Input: part model. Units: mm. Frame: model coordinates. A direction names the side the tool comes from. Round coordinates to 2 decimals unless told otherwise and drop trailing zeros. Loops run counter-clockwise (first coordinate to the right, second up) from the corner with the lowest first, then second, coordinate; pieces in that order, holes last.
(1) Cut plane D-D, the plane z = 18. Output: boundary loops of the cut face in (x, y), and give its area (3 significant figures).
(2) Access query for faces 4 (the face through (-55, 114, 0)), 5 (the face through (1.352, 222.535, 4.292)), 6 (the face through (-1, 220, 6)). Directions: +Z, -Z, +X, -X, +Y, -Y. A direction counts if a zero-diameter tool reaches every point of the face in a straight line with its end or side. Return the directions, or none.
(3) Cut plane B-B, the plane x = -68. Output: boundary loops of the cut face in (y, z).
(4) Cut plane A-A, the plane y = 135.5. Output: boundary loops of the cut face in (x, z).
(5) Line query: line 1 (X direction, y = 81, z = -1.5); line 2 (X direction, y = 222, z = 0); line 3 (Z direction, x = 68, y = 3.5). Output: solid intervals per line, ascending.
(6) Draft query along X for faces 1 (the face through (-63, 0, 0)), 2 (the face through (55, 111, 0)), 3 (the face through (-51.804, 1.711, 0.35)). Return one class per face: released by +X, released by -X, zero draft, split by the parting line, or undercut.
(7) First-contact query: pin 1 Ø25 at (y, z) = (92.5, -3) entering from -X; pin 2 Ø4 at (y, z) = (88, -11) entering from +X; pin 3 Ø19 at (x, z) = (64, 12.5) entering from +Y; pin 4 Ø8 at (x, z) = (68, 0) entering from -Y. Flat tips, straight axial feed; report the tip coordinate or a pass-through.
(8) Cut plane C-C, the plane z = 0. Give the number of separate pieces and of enclosed holes in the cut face, and give its area (3 significant figures).
from build123d import *

# Parameters (mm, degrees)
BASE_FLANGE1_DEPTH = 25
CUT_EXTRUDE1_REACH = 237.425
SKETCH7_R          = 3
CUT_EXTRUDE2_REACH = 242.104
SKETCH8_R          = 4.5
FILLET1_R          = 3


# Sheet-metal steps are written as plain solids
with BuildPart() as part:
    # Sketch1 → Base-Flange1 (new, symmetric)
    with BuildSketch(Plane.XY):
        with BuildLine():
            Line((-80, 0), (-56, 0))
            ThreePointArc((-56, 0), (-51.757359313, 1.757359313), (-50, 6))
            Line((-50, 6), (-50, 219))
            ThreePointArc((-50, 219), (-49.707106781, 219.707106781), (-49, 220))
            Line((-49, 220), (49, 220))
            ThreePointArc((49, 220), (49.707106781, 219.707106781), (50, 219))
            Line((50, 219), (50, 6))
            ThreePointArc((50, 6), (51.757359313, 1.757359313), (56, 0))
            Line((56, 0), (80, 0))
            Line((80, 0), (80, 5))
            Line((80, 5), (56, 5))
            ThreePointArc((56, 5), (55.292893219, 5.292893219), (55, 6))
            Line((55, 6), (55, 219))
            ThreePointArc((55, 219), (53.242640687, 223.242640687), (49, 225))
            Line((49, 225), (-49, 225))
            ThreePointArc((-49, 225), (-53.242640687, 223.242640687), (-55, 219))
            Line((-55, 219), (-55, 6))
            ThreePointArc((-55, 6), (-55.292893219, 5.292893219), (-56, 5))
            Line((-56, 5), (-80, 5))
            Line((-80, 5), (-80, 0))
        make_face()
    extrude(amount=BASE_FLANGE1_DEPTH, both=True)

    # Sketch7 → Cut-Extrude1 (cut, up to next)
    with BuildSketch(Plane(origin=(0, 5, 0), x_dir=(1, 0, 0), z_dir=(0, 1, 0)), mode=Mode.PRIVATE) as cut_extrude1_sk1:
        with Locations(Location((68, 0, 0), (0, 0, 180))):
            Circle(SKETCH7_R)
    cut_extrude1_tool1 = extrude(cut_extrude1_sk1.sketch, amount=-CUT_EXTRUDE1_REACH, mode=Mode.PRIVATE) & part.part
    # Sketch7 → Cut-Extrude1 (cut, up to next)
    with BuildSketch(Plane(origin=(0, 5, 0), x_dir=(1, 0, 0), z_dir=(0, 1, 0)), mode=Mode.PRIVATE) as cut_extrude1_sk2:
        with Locations(Location((-68, 0, 0), (0, 0, 180))):
            Circle(SKETCH7_R)
    cut_extrude1_tool2 = extrude(cut_extrude1_sk2.sketch, amount=-CUT_EXTRUDE1_REACH, mode=Mode.PRIVATE) & part.part
    add(cut_extrude1_tool1.solids().sort_by_distance((68, 5, 0))[0], mode=Mode.SUBTRACT)
    add(cut_extrude1_tool2.solids().sort_by_distance((-68, 5, 0))[0], mode=Mode.SUBTRACT)

    # Sketch8 → Cut-Extrude2 (cut, up to next)
    with BuildSketch(Plane(origin=(0, 225, 0), x_dir=(1, 0, 0), z_dir=(0, 1, 0)), mode=Mode.PRIVATE) as cut_extrude2_sk1:
        with Locations(Location((0, 0, 0), (0, 0, 270))):
            Circle(SKETCH8_R)
    cut_extrude2_tool1 = extrude(cut_extrude2_sk1.sketch, amount=-CUT_EXTRUDE2_REACH, mode=Mode.PRIVATE) & part.part
    # Sketch8 → Cut-Extrude2 (cut, up to next)
    with BuildSketch(Plane(origin=(0, 225, 0), x_dir=(1, 0, 0), z_dir=(0, 1, 0)), mode=Mode.PRIVATE) as cut_extrude2_sk2:
        with Locations(Location((-25, 0, 0), (0, 0, 270))):
            Circle(SKETCH8_R)
    cut_extrude2_tool2 = extrude(cut_extrude2_sk2.sketch, amount=-CUT_EXTRUDE2_REACH, mode=Mode.PRIVATE) & part.part
    # Sketch8 → Cut-Extrude2 (cut, up to next)
    with BuildSketch(Plane(origin=(0, 225, 0), x_dir=(1, 0, 0), z_dir=(0, 1, 0)), mode=Mode.PRIVATE) as cut_extrude2_sk3:
        with Locations(Location((25, 0, 0), (0, 0, 270))):
            Circle(SKETCH8_R)
    cut_extrude2_tool3 = extrude(cut_extrude2_sk3.sketch, amount=-CUT_EXTRUDE2_REACH, mode=Mode.PRIVATE) & part.part
    add(cut_extrude2_tool1.solids().sort_by_distance((0, 225, 0))[0], mode=Mode.SUBTRACT)
    add(cut_extrude2_tool2.solids().sort_by_distance((-25, 225, 0))[0], mode=Mode.SUBTRACT)
    add(cut_extrude2_tool3.solids().sort_by_distance((25, 225, 0))[0], mode=Mode.SUBTRACT)

    # Fillet1
    fillet1_edges = [part.edges().sort_by_distance(p)[0] for p in [
        (80, 2.5, -25),
        (-80, 2.5, -25),
        (80, 2.5, 25),
        (-80, 2.5, 25),
    ]]
    fillet(fillet1_edges, radius=FILLET1_R)


solid = part.part
Reported:
1. outline: (-80, 0) - (-56, 0) arc R6 ccw to (-50, 6) - (-50, 219) arc R1 cw to (-49, 220) - (49, 220) arc R1 cw to (50, 219) - (50, 6) arc R6 ccw to (56, 0) - (80, 0) - (80, 5) - (56, 5) arc R1 cw to (55, 6) - (55, 219) arc R6 ccw to (49, 225) - (-49, 225) arc R6 ccw to (-55, 219) - (-55, 6) arc R1 cw to (-56, 5) - (-80, 5) - close
1. area: 2,970 mm2
2. face 4: +Z, -Z, -X, +Y
2. face 5: +Y, -Y
2. face 6: +Z, -Z, -Y
3. outline: (0, -25) - (5, -25) - (5, -3) - (0, -3) - close; (0, 3) - (5, 3) - (5, 25) - (0, 25) - close
4. outline: (-55, -25) - (-50, -25) - (-50, 25) - (-55, 25) - close; (50, -25) - (55, -25) - (55, 25) - (50, 25) - close
5. line 1: x = -55 to -50, 50 to 55
5. line 2: x = -54.2 to -29.5, -20.5 to -4.5, 4.5 to 20.5, 29.5 to 54.2
5. line 3: z = -25 to -3, 3 to 25
6. face 1: zero draft
6. face 2: released by +X
6. face 3: undercut
7. pin 1: stops at x = -55
7. pin 2: stops at x = 55
7. pin 3: stops at y = 221.4
7. pin 4: stops at y = 0
8. separate pieces: 6
8. enclosed holes: 0
8. area: 2,770 mm2
